Model file for the job. Use its own axes, mm. Face numbers are marked on the shaded views. A direction names the side the tool comes from. Round coordinates to 2 decimals unless told otherwise and drop trailing zeros. Loops run counter-clockwise (first coordinate to the right, second up) from the corner with the lowest first, then second, coordinate; pieces in that order, holes last. Notation, with made-up numbers: (33, 67) - (92, 67) arc R30 cw to (92, 90) - close; hole circle Ø10 at (65.5, -1.5). An arc over 180 degrees is marked (long way). Use one line per item in the form item = value.
from build123d import *

# Parameters (mm, degrees)
SKETCH1_R           = 3
BOSS_EXTRUDE1_DEPTH = 10
CUT_EXTRUDE1_DEPTH  = 6
BOSS_EXTRUDE2_DEPTH = 10


with BuildPart() as part:
    # Sketch1 → Boss-Extrude1 (new body)
    with BuildSketch(Plane.XY):
        with BuildLine():
            Line((-5, 10), (10.134969828, 10))
            ThreePointArc((10.134969828, 10), (11.498966548, 9.462707403), (12.130097928, 8.139512947))
            Line((12.130097928, 8.139512947), (12.279025895, 6.009743799))
            Line((12.279025895, 6.009743799), (122.011071424, 13.682955911))
            Line((122.011071424, 13.682955911), (122.011071424, 15.827693331))
            ThreePointArc((122.011071424, 15.827693331), (122.54836402, 17.191690051), (123.871558476, 17.822821431))
            Line((123.871558476, 17.822821431), (127.996455725, 18.111262346))
            ThreePointArc((127.996455725, 18.111262346), (129.448086731, 17.625553406), (130.131096773, 16.255647193))
            Line((130.131096773, 16.255647193), (130.513028814, 10.79376454))
            ThreePointArc((130.513028814, 10.79376454), (129.45752894, 7.356802052), (126.3687377, 5.516649939))
            Line((126.3687377, 5.516649939), (12, -14.058605554))
            Line((12, -14.058605554), (12, -21))
            ThreePointArc((12, -21), (10.535533906, -24.535533906), (7, -26))
            Line((7, -26), (-5, -26))
            ThreePointArc((-5, -26), (-8.535533906, -24.535533906), (-10, -21))
            Line((-10, -21), (-10, 5))
            ThreePointArc((-10, 5), (-8.535533906, 8.535533906), (-5, 10))
        make_face()
        Circle(SKETCH1_R, mode=Mode.SUBTRACT)
        with Locations((0, -18)):
            Circle(SKETCH1_R, mode=Mode.SUBTRACT)
    extrude(amount=BOSS_EXTRUDE1_DEPTH)

    # Sketch2 → Cut-Extrude1 (cut)
    with BuildSketch(Plane.XY.offset(10)):
        with BuildLine():
            Line((12, -5.257633034), (12, -1.749595529))
            ThreePointArc((12, -1.749595529), (13.074585194, 0.978397911), (15.720974105, 2.240660672))
            Line((15.720974105, 2.240660672), (100.359457674, 8.159159996))
            ThreePointArc((100.359457674, 8.159159996), (101.953365437, 6.84188311), (100.717151126, 5.18431425))
            Line((100.717151126, 5.18431425), (16.67482331, -9.20029882))
            ThreePointArc((16.67482331, -9.20029882), (13.421172092, -8.31535222), (12, -5.257633034))
        make_face()
    extrude(amount=-CUT_EXTRUDE1_DEPTH, mode=Mode.SUBTRACT)

    # Sketch4 → Boss-Extrude2 (add)
    with BuildSketch(Plane.XY.offset(10)):
        Polygon((12, -18.990256201), (48, -7.896876292), (12, -14.058605554), align=None)
    extrude(amount=-BOSS_EXTRUDE2_DEPTH)


solid = part.part
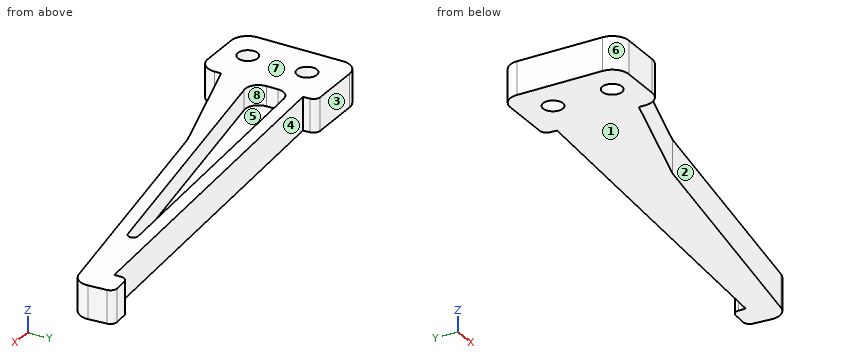
1. Wall check: probe 1 along Y at (x, z) = (0, 3.75); probe 2 along Z at (x, y) = (23, -8); probe 3 along Y at (x, z) = (78.5, 5.5). Give the ranges that are in metal, low to high.
Geometry check:
probe_1 = -26 to -21, -15 to -3, 3 to 10
probe_2 = 0 to 4
probe_3 = -2.68 to 1.38, 6.63 to 10.64
2. Cut at B-B, the plane x = 0. Give the cut face in (y, z), plus the area to 3 significant figures.
Geometry check:
outline = (-26, 0) - (-21, 0) - (-21, 10) - (-26, 10) - close; (-15, 0) - (-3, 0) - (-3, 10) - (-15, 10) - close; (3, 0) - (10, 0) - (10, 10) - (3, 10) - close
area = 240 mm^2
3. Cut at A-A, the plane z = 1.75. Give the cut face in (x, y), plus the area to 3 significant figures.
Geometry check:
outline = (-10, -21) arc R5 ccw to (-5, -26) - (7, -26) arc R5 ccw to (12, -21) - (12, -18.99) - (48, -7.9) - (126.37, 5.52) arc R5 ccw to (130.51, 10.79) - (130.13, 16.26) arc R2 ccw to (128, 18.11) - (123.87, 17.82) arc R2 ccw to (122.01, 15.83) - (122.01, 13.68) - (12.28, 6.01) - (12.13, 8.14) arc R2 ccw to (10.13, 10) - (-5, 10) arc R5 ccw to (-10, 5) - close; hole circle Ø6 at (0, -18); hole circle Ø6 at (0, 0)
area = 2,500 mm^2
4. Pull direction Y, two halves, no side cores. Call the marked faces 6, 7 and 8: +Y half, -Y half, draft (parallel to the pull), parting line (faces both ways), or undercut.
Geometry check:
face_6 = -Y half
face_7 = draft
face_8 = undercut
5. Flat gauge pins, fed straight in: pin 1 (1 mm diameter, centred on x = 90, z = 5, fed in from +Y); pin 2 (1.5 mm diameter, centred on x = 24.5, z = 1.5, fed in from +Y); pin 3 (1 mm diameter, centred on x = 114, z = 3.5, fed in from -Y). Where does each tip first touch, or does it go through?
Geometry check:
pin_1 = 11.48
pin_2 = 6.92
pin_3 = 3.31
6. Tool access for the marked faces 1, 2, 3, 4 and 5: list every direction of +Z, -Z, +X, -X, +Y, -Y with a clear straight run to the whole face (end or side of a thin tool).
Geometry check:
face_1 = -Z, +X, -X, +Y, -Y
face_2 = +Z, -Z, +X, -Y
face_3 = +Z, -Z, -X, +Y
face_4 = +Z, -Z, +Y
face_5 = +Z
7. Cut at C-C, the plane y = 0. Give the cut face in (x, z).
Geometry check:
outline = (-10, 0) - (-3, 0) - (-3, 10) - (-10, 10) - close; (3, 0) - (94.14, 0) - (94.14, 10) - (70.43, 10) - (70.43, 4) - (12.4, 4) - (12.4, 10) - (3, 10) - close
8. Cut at D-D, the plane x = 116. Give the cut face in (y, z).
Geometry check:
outline = (3.74, 0) - (13.26, 0) - (13.26, 10) - (3.74, 10) - close
